```python
from build123d import *

# Parameters (mm, degrees)
F0_W     = 23.7744
F0_H     = 7.7978
F1_DEPTH = 4.7879
F2_R     = 2.4511
F3_DEPTH = 1.8288
F4_W     = 20.7264
F4_H     = 4.7498
F6_DEPTH = 8.0772
F5_R     = 1.4859
F5_R_2   = 1.5621
F7_DEPTH = 8.0772


with BuildPart() as f1:
    # F0 (on Top) → F1 (new body, symmetric)
    with BuildSketch(Plane.XY):
        Rectangle(F0_W, F0_H)
    extrude(amount=F1_DEPTH, both=True)

    # F2 (on face) → F3 (join)
    with BuildSketch(Plane.XY.offset(4.7879)):
        with Locations((-7.9756, 0)):
            Circle(F2_R)
        Circle(F2_R)
        with Locations((7.9756, 0)):
            Circle(F2_R)
    extrude(amount=F3_DEPTH)

    # F4 (on face) → F6 (cut)
    with BuildSketch(Plane(origin=(0, 0, -4.7879), x_dir=(1, 0, 0), z_dir=(0, 0, -1))):
        Rectangle(F4_W, F4_H)
    extrude(amount=-F6_DEPTH, mode=Mode.SUBTRACT)

    # F5 (on face) → F7 (join)
    with BuildSketch(Plane(origin=(0, 0, -4.7879), x_dir=(1, 0, 0), z_dir=(0, 0, -1))):
        with Locations((-4.0005, 0)):
            Circle(F5_R)
        with Locations((3.9243, 0)):
            Circle(F5_R_2)
    extrude(amount=-F7_DEPTH)


solid = f1.part
```
Build history of the part. All positions in model axes, mm. A direction names the side the tool comes from. Round coordinates to 2 decimals unless told otherwise and drop trailing zeros. Write each loop counter-clockwise with the first axis right and the second up, starting at its lowest first coordinate (ties: lowest second). Pieces come first, ordered by that corner, then holes. Notation, with made-up numbers: (-30.5, 31.5) - (12.5, 31.5) arc R15 cw to (12.5, 45.5) - close; hole circle Ø6 at (76, -38.5). An arc over 180 degrees is marked (long way). Answer as CSV lines item,"result".
Q1. Drop a flat-ended pin along its axis: pin 1 (2 mm diameter, centred on x = 7, y = -0.5, fed in from -Z). Give the stop position or say it passes through.
Report:
pin 1,"stops at z = 3.29"
Q2. Cut at A-A (z = -3.75). Write the cut outline in (x, y).
Report:
outline,"(-11.89, -3.9) - (11.89, -3.9) - (11.89, 3.9) - (-11.89, 3.9) - close; circle Ø2.97 at (-4, 0); circle Ø3.12 at (3.92, 0); hole (-10.36, -2.37) - (10.36, -2.37) - (10.36, 2.37) - (-10.36, 2.37) - close"
Q3. Pull direction X, two halves, no side cores. Call faces 1 (the flat face through (-11.887, 0, 0)), 2 (the flat face through (0, 2.375, -1)), 3 (the flat face through (8, 0, 6.617)): +X half, -X half, draft (parallel to the pull), parting line (faces both ways), or undercut.
Report:
face 1,"-X half"
face 2,"undercut"
face 3,"draft"
Q4. Cut at B-B (x = 0). Write the cut outline in (y, z), and give its area (3 significant figures).
Report:
outline,"(-3.9, -4.79) - (-2.37, -4.79) - (-2.37, 3.29) - (2.37, 3.29) - (2.37, -4.79) - (3.9, -4.79) - (3.9, 4.79) - (2.45, 4.79) - (2.45, 6.62) - (-2.45, 6.62) - (-2.45, 4.79) - (-3.9, 4.79) - close"
area,"45.3 mm^2"
Q5. Drill centre lines: probe 1 along Y at (x, z) = (-4, 0.75); probe 2 along Y at (x, z) = (8, -4); probe 3 along X at (y, z) = (-2, 5). Where is each one in solid material? Low to high. Write a range as [from, to].
Report:
probe 1,"y = [-3.9, -2.37], [-1.49, 1.49], [2.37, 3.9]"
probe 2,"y = [-3.9, -2.37], [2.37, 3.9]"
probe 3,"x = [-9.39, -6.56], [-1.42, 1.42], [6.56, 9.39]"
Q6. Tool access for faces 4 (the cylindrical face through (2.338, 0.736, 5.689)), 5 (the flat face through (10.363, 0, -1)), 6 (the flat face through (11.887, 0, 0)): list every direction of +Z, -Z, +X, -X, +Y, -Y with a clear straight run to the whole face (end or side of a thin tool).
Report:
face 4,"+Z"
face 5,"-Z"
face 6,"+Z, -Z, +X, +Y, -Y"
Q7. Cut at C-C (y = 0). Write the cut outline in (x, z).
Report:
outline,"(-11.89, -4.79) - (-10.36, -4.79) - (-10.36, 3.29) - (-5.49, 3.29) - (-5.49, -4.79) - (-2.51, -4.79) - (-2.51, 3.29) - (2.36, 3.29) - (2.36, -4.79) - (5.49, -4.79) - (5.49, 3.29) - (10.36, 3.29) - (10.36, -4.79) - (11.89, -4.79) - (11.89, 4.79) - (10.43, 4.79) - (10.43, 6.62) - (5.52, 6.62) - (5.52, 4.79) - (2.45, 4.79) - (2.45, 6.62) - (-2.45, 6.62) - (-2.45, 4.79) - (-5.52, 4.79) - (-5.52, 6.62) - (-10.43, 6.62) - (-10.43, 4.79) - (-11.89, 4.79) - close"
Q8. Cut at D-D (x = 5.25). Write the cut outline in (y, z).
Report:
outline,"(-3.9, -4.79) - (-2.37, -4.79) - (-2.37, 3.29) - (-0.83, 3.29) - (-0.83, -4.79) - (0.83, -4.79) - (0.83, 3.29) - (2.37, 3.29) - (2.37, -4.79) - (3.9, -4.79) - (3.9, 4.79) - (-3.9, 4.79) - close"
